CAD build for the part. Positions are in the model's coordinates, mm. Face numbers are marked on the shaded views. Coordinates: 2 decimals unless noted, no trailing zeros. Write each loop counter-clockwise with the first axis right and the second up, starting at its lowest first coordinate (ties: lowest second). Pieces come first, ordered by that corner, then holes. Notation, with made-up numbers: (-2.75, 8) -> (45.25, 8) arc R17 cw to (45.25, 15) -> close; hole circle Ø11 at (-6.5, -38.5). An arc over 180 degrees is marked (long way). Answer as CSV lines item,"result".
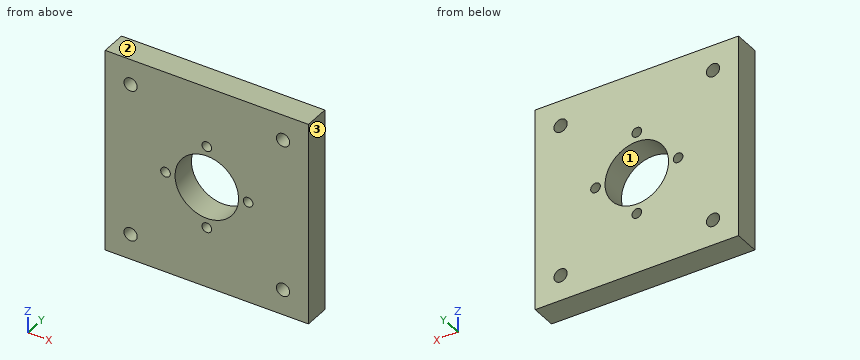
```python
from build123d import *

# Parameters (mm, degrees)
SKETCH2_W           = 101.6
SKETCH2_H           = 101.6
BOSS_EXTRUDE1_DEPTH = 6.35
SKETCH3_R           = 3.302
CUT_EXTRUDE1_DEPTH  = 73.955945611
SKETCH4_R           = 15.875
SKETCH4_R_2         = 2.413
CUT_EXTRUDE2_DEPTH  = 73.955945611


with BuildPart() as part:
    # Sketch2 → Boss-Extrude1 (new, symmetric)
    with BuildSketch(Plane(origin=(0, 0, 0), x_dir=(1, 0, 0), z_dir=(0, 1, 0))):
        Rectangle(SKETCH2_W, SKETCH2_H)
    extrude(amount=BOSS_EXTRUDE1_DEPTH, both=True)

    # Sketch3 → Cut-Extrude1 (cut, through all)
    with BuildSketch(Plane(origin=(0, 6.35, 0), x_dir=(1, 0, 0), z_dir=(0, 1, 0))):
        with Locations(Location((-38.1, -38.1, 0), (0, 0, 270))):
            Circle(SKETCH3_R)
        with Locations(Location((-38.1, 38.1, 0), (0, 0, 90))):
            Circle(SKETCH3_R)
        with Locations(Location((38.1, -38.1, 0), (0, 0, 90))):
            Circle(SKETCH3_R)
        with Locations(Location((38.1, 38.1, 0), (0, 0, 270))):
            Circle(SKETCH3_R)
    extrude(amount=-CUT_EXTRUDE1_DEPTH, mode=Mode.SUBTRACT)

    # Sketch4 → Cut-Extrude2 (cut, through all)
    with BuildSketch(Plane(origin=(0, 6.35, 0), x_dir=(1, 0, 0), z_dir=(0, 1, 0))):
        with Locations(Location((0, 0, 0), (0, 0, 270))):
            Circle(SKETCH4_R)
        with Locations(Location((0, 20.6375, 0), (0, 0, 270))):
            Circle(SKETCH4_R_2)
        with Locations(Location((20.6375, 0, 0), (0, 0, 270))):
            Circle(SKETCH4_R_2)
        with Locations(Location((0, -20.6375, 0), (0, 0, 270))):
            Circle(SKETCH4_R_2)
        with Locations(Location((-20.6375, 0, 0), (0, 0, 270))):
            Circle(SKETCH4_R_2)
    extrude(amount=-CUT_EXTRUDE2_DEPTH, mode=Mode.SUBTRACT)


solid = part.part
```
Item 1: Saw through at A-A on x = 38.1. Give the cut face in (y, z), and give its area (3 significant figures).
Answer below:
outline,"(-6.35, -50.8) -> (6.35, -50.8) -> (6.35, -41.4) -> (-6.35, -41.4) -> close; (-6.35, -34.8) -> (6.35, -34.8) -> (6.35, 34.8) -> (-6.35, 34.8) -> close; (-6.35, 41.4) -> (6.35, 41.4) -> (6.35, 50.8) -> (-6.35, 50.8) -> close"
area,"1,120 mm2"
Item 2: Flat gauge pin, fed straight in: pin 1 (6 mm diameter, centred on x = -12.5, z = 6.5, fed in from +Y). Where does the tip first touch, or does it go through?
Answer below:
pin 1,"stops at y = 6.35"
Item 3: Wall check: line 1 (X direction, y = -1.75, z = 38.1); line 2 (Z direction, x = -40, y = 2.25); line 3 (Z direction, x = 41, y = 0.5). Give the ranges that are in metal, low to high. Write a range as from..to.
Answer below:
line 1,"x = -50.8..-41.4, -34.8..34.8, 41.4..50.8"
line 2,"z = -50.8..-40.8, -35.4..35.4, 40.8..50.8"
line 3,"z = -50.8..-39.68, -36.52..36.52, 39.68..50.8"
Item 4: Saw through at B-B on z = 0. State how many separate pieces and enclosed holes the cut face has, and give its area (3 significant figures).
Answer below:
separate pieces,"4"
enclosed holes,"0"
area,"765 mm2"
Item 5: Saw through at C-C on z = -38.1. Give the cut face in (x, y).
Answer below:
outline,"(-50.8, -6.35) -> (-41.4, -6.35) -> (-41.4, 6.35) -> (-50.8, 6.35) -> close; (-34.8, -6.35) -> (34.8, -6.35) -> (34.8, 6.35) -> (-34.8, 6.35) -> close; (41.4, -6.35) -> (50.8, -6.35) -> (50.8, 6.35) -> (41.4, 6.35) -> close"
Item 6: Two-plate mould, pull along Z, no slides. Class the marked faces 1, 2 and 3: pulls with the +Z half, pulls with the -Z half, needs draft (parallel to the pull), parting line crosses it, or undercut.
Answer below:
face 1,"undercut"
face 2,"pulls with the +Z half"
face 3,"needs draft"
